Solid Edge part; units mm, degrees
sketch "Sketch1" plane through (0, 0, 0) normal (0, 0, 1) x (1, 0, 0)
  line L0 (0, 0) -> (0, 10)
  line L1 (0, 10) -> (64.8, 10)
  line L2 (64.8, 10) -> (64.8, -10)
  line L3 (64.8, -10) -> (0, -10)
  line L4 (0, -10) -> (0, 0)
extrude "Protrusion1" add sketch "Sketch1" against normal blind 10
sketch "Sketch2" plane through (32.4, 0, 0) normal (0, 0, 1) x (1, 0, 0)
  circle A0 centre (-32.4, -6.1) radius 6.5
extrude "Recorte_Extrudado_1" cut sketch "Sketch2" against normal blind 10
sketch "Sketch3" plane through (32.4, 0, 0) normal (0, 0, 1) x (-1, 0, 0)
  circle A0 centre (32.4, 6.1) radius 14
extrude "Recorte_Extrudado_2" cut sketch "Sketch3" against normal blind 3
sketch "Sketch4" plane through (32.4, 0, 0) normal (0, 0, 1) x (1, 0, 0)
  line L0 (-27.2, -10) -> (-27.2, -7.6)
  line L1 (-19.5, -10) -> (-27.2, -7.6)
  line L2 (-27.2, -10) -> (-19.5, -10)
extrude "Recorte_Extrudado_3" cut sketch "Sketch4" against normal blind 10
For this review, take the finished solid that the model builds, in its own axes (mm). A direction names the side the tool comes from. Coordinates: 2 decimals unless noted, no trailing zeros. Loops run counter-clockwise (first coordinate to the right, second up) from the corner with the lowest first, then second, coordinate; pieces in that order, holes last. Notation, with made-up numbers: (-10.75, 27) - (24.25, 27) arc R12 ccw to (24.25, 45) - close; hole circle Ø7 at (1.25, 65.5). An arc over 180 degrees is marked (long way). Use one line per item in the form item = value. Start each with the question number.
1) To check wall thickness, follow probe 1 along Z at (x, y) = (9, 3.25); probe 2 along X at (y, z) = (-3, -5.5); probe 3 along Y at (x, z) = (11, -7.25). State the ranges of each line that lie inside material, in increasing order. Write a range as from..to.
2) Take a section at A-A (z = -7). State the section outline as (x, y) points.
3) Take a section at C-C (z = -2.25). State the section outline as (x, y) points.
4) Take a section at B-B (y = 4.25). State the section outline as (x, z) points.
5) For faces 1 (the face through (11.302, 2.162, -1.479)), 2 (the face through (32, 10, -5)), list the 3-axis set-ups (+Z, -Z, +X, -X, +Y, -Y) from which the entire face can be reached by the end or side of a thin tool; tool diameter is ignored.
6) For pin 1 (4 mm diameter, centred on x = 10, z = -6.5, fed in from -Y), flat-tipped, find the tip position at first contact; note if it passes through.
From the geometry:
q1.probe_1 = -10..-3
q1.probe_2 = 5.71..64.8
q1.probe_3 = -9.41..10
q2.outline = (0, 0.4) arc R6.5 cw to (6.24, -7.92) - (12.9, -10) - (64.8, -10) - (64.8, 10) - (0, 10) - close
q3.outline = (0, 7.9) arc R14 cw to (13.45, -10) - (64.8, -10) - (64.8, 10) - (0, 10) - close
q4.outline = (0, -10) - (64.8, -10) - (64.8, 0) - (9.43, 0) - (9.43, -3) - (0, -3) - close
q5.face_1 = +Z, -X
q5.face_2 = +Z, -Z, +X, -X, +Y
q6.pin_1 = -9.72
